Verification items for the finished model (mm, model axes). A direction names the side the tool comes from. Give positions to 0.01 mm unless a question says otherwise; leave off trailing zeros. Loops run counter-clockwise (first coordinate to the right, second up) from the corner with the lowest first, then second, coordinate; pieces in that order, holes last. Notation, with made-up numbers: M -31,80.25 L -4,80.25 A18 ccw -4,84.25 Z; hole C 44,44 d4. An arc over 180 degrees is marked long. Put each result on its own line as item: value. Start each with the question number.
from build123d import *

# Parameters (mm, degrees)
SKETCH2_R          = 9.53135
CUT_EXTRUDE1_DEPTH = 29.575


with BuildPart() as part:
    # Sketch1 → Revolve1 (revolve)
    with BuildSketch(Plane.XY, mode=Mode.PRIVATE) as revolve1_sk:
        with BuildLine():
            Line((-14.2875, 0), (14.2875, 0))
            Line((14.2875, 0), (14.2875, 57.793141026))
            Line((14.2875, 57.793141026), (13.49375, 58.586891026))
            Line((13.49375, 58.586891026), (6.659344616, 58.586891026))
            ThreePointArc((6.659344616, 58.586891026), (5.778331049, 58.274323253), (5.291300439, 57.476398003))
            Line((5.291300439, 57.476398003), (3.883957867, 50.777754993))
            ThreePointArc((3.883957867, 50.777754993), (0, 47.625), (-3.883957867, 50.777754993))
            Line((-3.883957867, 50.777754993), (-5.291300439, 57.476398003))
            ThreePointArc((-5.291300439, 57.476398003), (-5.778331049, 58.274323253), (-6.659344616, 58.586891026))
            Line((-6.659344616, 58.586891026), (-13.49375, 58.586891026))
            Line((-13.49375, 58.586891026), (-14.2875, 57.793141026))
            Line((-14.2875, 57.793141026), (-14.2875, 0))
        make_face()
    revolve(revolve1_sk.sketch.rotate(Axis((-14.2875, 0, 0), (1, 0, 0)), 90), axis=Axis((-14.2875, 0, 0), (1, 0, 0)))  # turned: the seam where the file's is

    # Sketch2 → Cut-Extrude1 (cut, through all)
    with BuildSketch(Plane(origin=(14.2875, 0, 0), x_dir=(0, 0, -1), z_dir=(1, 0, 0))):
        Circle(SKETCH2_R)
    extrude(amount=-CUT_EXTRUDE1_DEPTH, mode=Mode.SUBTRACT)


solid = part.part
Q1. Release check for a two-part mould opening along Z. For faces 1 (the face through (-14.288, -1, 12)), 2 (the face through (0.2, 9.45, 1.24)), 3 (the face through (10.029, 57.194, -12.7)) record: pulls with the +Z half, pulls with the -Z half, needs draft (parallel to the pull), parting line crosses it, or undercut.
Q2. Set-up check for faces 4 (the face through (3.952, 49.888, -11.078)), 5 (the face through (-10.124, 57.194, -12.7)): record each of +Z, -Z, +X, -X, +Y, -Y from which the full face is reachable in a straight line by a thin tool's end or side.
Q3. Scan lines: L1, parallel to X at y = 50, z = 9; L2, parallel to Y at x = -3, z = 0; L3, parallel to X at y = -50, z = -22.5. Record each from-to range of solid material in increasing order.
Q4. Cross-section at C-C, the plane x = -10.5. Record the boundary of the cut face in (y, z).
Q5. Cross-section at A-A, the plane z = 0. Record the boundary of the cut face in (x, y).
Q6. Go/stop test with flat-tipped pins: pin 1 (8 mm diameter, centred on x = 2, y = 13, fed in from +Z); pin 2 (1 mm diameter, centred on x = -7, y = 18.5, fed in from -Z); pin 3 (6 mm diameter, centred on x = -4, z = -21, fed in from +Y); pin 4 (15.5 mm diameter, centred on y = 0, z = 0, fed in from -X). Record where each tip stops, or that it passes through.
Ans:
1. face 1: needs draft
1. face 2: undercut
1. face 3: parting line crosses it
2. face 4: none
2. face 5: +X, -X
3. L1: x = -14.29 to -3.89, 3.89 to 14.29
3. L2: y = -49 to -9.53, 9.53 to 49
3. L3: x = -14.29 to -4.74, 4.74 to 14.29
4. outline: C 0,0 d117.17; hole C 0,0 d19.06
5. outline: M -14.29,-57.79 L -13.49,-58.59 L -6.66,-58.59 A1.4 ccw -5.29,-57.48 L -3.88,-50.78 A3.97 cw 3.88,-50.78 L 5.29,-57.48 A1.4 ccw 6.66,-58.59 L 13.49,-58.59 L 14.29,-57.79 L 14.29,-9.53 L -14.29,-9.53 Z; M -14.29,9.53 L 14.29,9.53 L 14.29,57.79 L 13.49,58.59 L 6.66,58.59 A1.4 ccw 5.29,57.48 L 3.88,50.78 A3.97 cw -3.88,50.78 L -5.29,57.48 A1.4 ccw -6.66,58.59 L -13.49,58.59 L -14.29,57.79 Z
6. pin 1: stops at z = 57.1
6. pin 2: stops at z = -55.75
6. pin 3: stops at y = 55.35
6. pin 4: passes through
